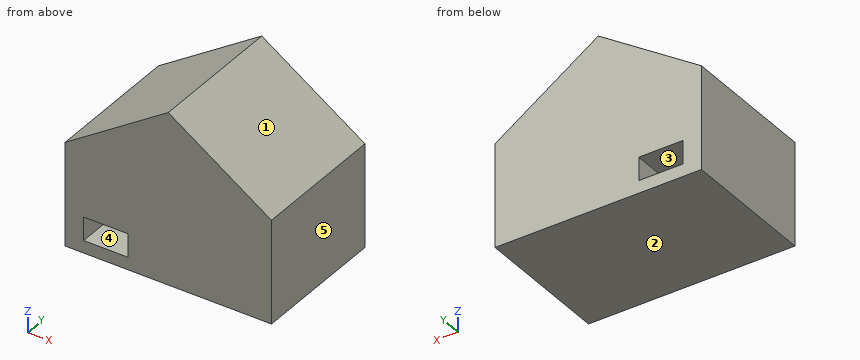
```python
from build123d import *

# Parameters (mm, degrees)
F0_W     = 32.065868
F0_H     = 16.976055
F0_W_2   = 15
F0_H_2   = 30
F1_DEPTH = 100


with BuildPart() as f1:
    # F0 (on Front) → F1 (new body)
    with BuildSketch(Plane.XZ):
        Polygon((-75, 0), (-75, -75), (-7.090706, -75), (-7.090706, -45), (7.909294, -45), (7.909294, -75), (75, -75), (75, 0), align=None)
        with Locations((-45.458086, -57.435633)):
            Rectangle(F0_W, F0_H, mode=Mode.SUBTRACT)
        Polygon((0, 49.749372), (-75, 0), (75, 0), align=None)
        with Locations((0.409294, -60)):
            Rectangle(F0_W_2, F0_H_2)
    extrude(amount=F1_DEPTH)


solid = f1.part
```
The model under review builds one solid part; all positions refer to its coordinate system, in mm. Face numbers are marked on the shaded views. A direction names the side the tool comes from. Round coordinates to 2 decimals unless told otherwise and drop trailing zeros. Loops run counter-clockwise (first coordinate to the right, second up) from the corner with the lowest first, then second, coordinate; pieces in that order, holes last. Notation, with made-up numbers: (-5, -28.5) -> (41, -28.5) arc R28 cw to (41, 8.5) -> close; hole circle Ø5 at (3, 89.25). An arc over 180 degrees is marked (long way). Answer as a JSON object with one key per item and string values. Group by question number.
1) For line 1 (Z direction, x = -41.5, y = -81.5); line 2 (Z direction, x = 49, y = -61); line 3 (Z direction, x = -31.5, y = -13.5), list the stretches that pass through material, from the lowest coordinate up. Write a range as [from, to].
2) We need section A-A on z = -53. Write out the cut boundary in (x, y), then the cut area to 3 significant figures.
3) We need section D-D on x = -23. Write out the cut boundary in (y, z), then the cut area to 3 significant figures.
4) For pin 1 Ø1.5 at (x, z) = (26.5, -39) entering from +Y; pin 2 Ø1 at (y, z) = (-36.5, 4.5) entering from -X; pin 3 Ø6 at (y, z) = (-55, 19.5) entering from -X, all flat-tipped, find the tip position at first contact; note any pin that passes through.
5) Mouldability with a two-part tool opening along X and no side actions: class the marked faces 1, 2 and 3 as released by +X, released by -X, zero draft, split by the parting line, or undercut.
6) We need section C-C on x = -45.5. Write out the cut boundary in (y, z), then the cut area to 3 significant figures.
7) We need section B-B on y = -85. Write out the cut boundary in (x, z).
8) For the marked faces 4 and 5, list the 3-axis set-ups (+Z, -Z, +X, -X, +Y, -Y) from which the entire face can be reached by the end or side of a thin tool; tool diameter is ignored.
Result set:
{
 "1": {"line 1": "[-75, -65.92], [-48.95, 22.22]", "line 2": "[-75, 17.25]", "line 3": "[-75, -65.92], [-48.95, 28.85]"},
 "2": {"outline": "(-75, -100) -> (-61.49, -100) -> (-61.49, 0) -> (-75, 0) -> close; (-29.43, -100) -> (75, -100) -> (75, 0) -> (-29.43, 0) -> close", "area": "11,800 mm²"},
 "3": {"outline": "(-100, -75) -> (0, -75) -> (0, 34.49) -> (-100, 34.49) -> close", "area": "10,900 mm²"},
 "4": {"pin 1": "y = 0", "pin 2": "x = -68.97", "pin 3": "x = -50.13"},
 "5": {"face 1": "released by +X", "face 2": "zero draft", "face 3": "undercut"},
 "6": {"outline": "(-100, -75) -> (0, -75) -> (0, -65.92) -> (-100, -65.92) -> close; (-100, -48.95) -> (0, -48.95) -> (0, 19.57) -> (-100, 19.57) -> close", "area": "7,760 mm²"},
 "7": {"outline": "(-75, -75) -> (75, -75) -> (75, 0) -> (0, 49.75) -> (-75, 0) -> close; hole (-61.49, -65.92) -> (-29.43, -65.92) -> (-29.43, -48.95) -> (-61.49, -48.95) -> close"},
 "8": {"face 4": "+Y, -Y", "face 5": "+Z, -Z, +X, +Y, -Y"}
}
